from build123d import *

# Parameters (mm, degrees)
SKETCH_1_R               = 8.5
EXTRUDE_1_DEPTH          = 1.2
SKETCH_2_R               = 8.5
SKETCH_2_R_2             = 7
EXTRUDE_2_DEPTH          = 5.5
SKETCH_3_R               = 7
SKETCH_3_R_2             = 6.5
EXTRUDE_3_DEPTH          = 0.3
SKETCH_4_W               = 1
SKETCH_4_H               = 4.082242853
CUT_EXTRUDE_1_DEPTH      = 5
PATTERN_CIRCULAR_1_COUNT = 8
SKETCH_5_W               = 1.4
SKETCH_5_H               = 2.4
EXTRUDE_4_DEPTH          = 1.7


with BuildPart() as part:
    # Эскиз1 → Бобышка-Вытянуть1 (new body)
    with BuildSketch(Plane(origin=(0, 0, 0), x_dir=(1, 0, 0), z_dir=(0, 1, 0))):
        with Locations(Location((0, 0, 0), (0, 0, 270))):
            Circle(SKETCH_1_R)
    extrude(amount=EXTRUDE_1_DEPTH)

    # Эскиз2 → Бобышка-Вытянуть2 (add)
    with BuildSketch(Plane(origin=(0, 1.2, 0), x_dir=(1, 0, 0), z_dir=(0, 1, 0))):
        with Locations(Location((0, 0, 0), (0, 0, 270))):
            Circle(SKETCH_2_R)
        with Locations(Location((0, 0, 0), (0, 0, 270))):
            Circle(SKETCH_2_R_2, mode=Mode.SUBTRACT)
    extrude(amount=EXTRUDE_2_DEPTH)

    # Эскиз3 → Бобышка-Вытянуть3 (add)
    with BuildSketch(Plane(origin=(0, 1.2, 0), x_dir=(1, 0, 0), z_dir=(0, 1, 0))):
        with Locations(Location((0, 0, 0), (0, 0, 270))):
            Circle(SKETCH_3_R)
        with Locations(Location((0, 0, 0), (0, 0, 270))):
            Circle(SKETCH_3_R_2, mode=Mode.SUBTRACT)
    extrude(amount=EXTRUDE_3_DEPTH)

    # Эскиз4 → Вырез-Вытянуть1 (cut)
    with BuildSketch(Plane(origin=(0, 6.7, 0), x_dir=(1, 0, 0), z_dir=(0, 1, 0))):
        with Locations((0, 7.692447021)):
            Rectangle(SKETCH_4_W, SKETCH_4_H)
    cut_extrude_1 = extrude(amount=-CUT_EXTRUDE_1_DEPTH, mode=Mode.SUBTRACT)

    # Круговой массив1: Вырез-Вытянуть1 ×8 about axis
    pattern_circular_1_axis = Axis((0, 0, 0), (0, 1, 0))
    for i in range(1, PATTERN_CIRCULAR_1_COUNT):
        add(cut_extrude_1.rotate(pattern_circular_1_axis, i * 360 / PATTERN_CIRCULAR_1_COUNT), mode=Mode.SUBTRACT)

    # Эскиз5 → Бобышка-Вытянуть4 (add)
    with BuildSketch(Plane.XZ):
        with BuildLine():
            Line((-11.124038405, -2.5), (-8.124038405, -2.5))
            ThreePointArc((-8.124038405, -2.5), (-8.5, 0), (-8.124038405, 2.5))
            Line((-8.124038405, 2.5), (-11.124038405, 2.5))
            ThreePointArc((-11.124038405, 2.5), (-11.831145186, 2.207106781), (-12.124038405, 1.5))
            Line((-12.124038405, 1.5), (-12.124038405, -1.5))
            ThreePointArc((-12.124038405, -1.5), (-11.831145186, -2.207106781), (-11.124038405, -2.5))
        make_face()
        with Locations((-10.124038405, 0)):
            Rectangle(SKETCH_5_W, SKETCH_5_H, mode=Mode.SUBTRACT)
    extrude(amount=-EXTRUDE_4_DEPTH)


solid = part.part
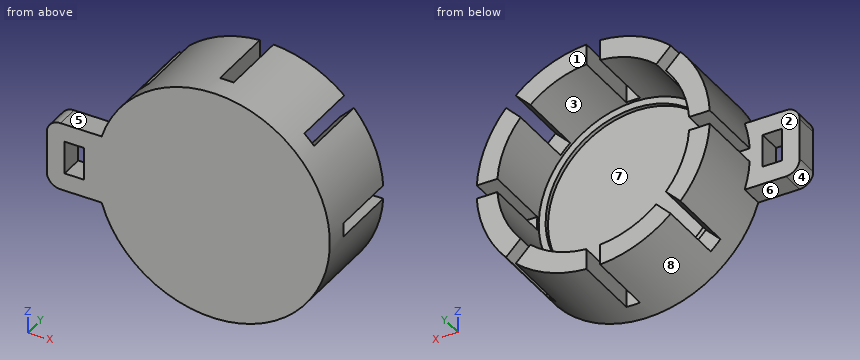
Read the model definition and answer for the solid it produces. Units are mm, in the model's axes. Face numbers are marked on the shaded views. A direction names the side the tool comes from. Give positions to 0.01 mm unless a question says otherwise; leave off trailing zeros. Write each loop counter-clockwise with the first axis right and the second up, starting at its lowest first coordinate (ties: lowest second). Pieces come first, ordered by that corner, then holes. Notation, with made-up numbers: (-34, -16.5) -> (-10, -16.5) arc R25 ccw to (-10, 3.5) -> close; hole circle Ø5 at (86.5, 8.5). An arc over 180 degrees is marked (long way). Answer as a JSON object with one key per item and string values. Group by question number.
1) The mould has two halves that part along X. Classify the marked faces 6, 7 and 8: +X half, -X half, draft (parallel to the pull), parting line (faces both ways), or undercut.
2) Consider L1, parallel to X at y = 1.4, z = 0; L2, parallel to Y at x = 2.25, z = -1.75; L3, parallel to X at y = 5, z = 5. Determine where each line is inside the solid, lowest interval first. Write a range as from..to.
3) Each of these flat-tipped pins is pushed along its axis until it touches: P1, Ø2, axis at x = -5.5, y = 0.5, coming from the +Z side; P2, Ø2, axis at x = -10, y = 2.5, coming from the +Z side; P3, Ø1.5, axis at x = -8, y = 3, coming from the +Z side; P4, Ø0.5, axis at x = 6, z = -5.5, coming from the +Y side. Where does it stop, or does it pass through?
4) Find section D-D (x = 0). Write down the section's boundary in (y, z), and give its area (3 significant figures).
5) Find section C-C (z = 0). Write down the section's boundary in (x, y).
6) A tool of negligible diameter and unlimited length cuts with its end or side. For the marked faces 1, 2, 3, 4 and 5, from which of +Z, -Z, +X, -X, +Y, -Y can it reach the whole face along a straight path? Write none if from no direction.
7) Find section B-B (x = -10.5). Write down the section's boundary in (y, z).
8) Find section A-A (y = 3.5). Count the separate pieces of the cut face and the enclosed holes in it, and give its area (3 significant figures).
Values follow:
{
 "1": {"face 6": "draft", "face 7": "undercut", "face 8": "parting line"},
 "2": {"L1": "x = -12.12..-10.82, -9.42..-6.5, 6.5..8.5", "L2": "y = 0..1.2", "L3": "x = -6.87..-5.71, 5.71..6.87"},
 "3": {"P1": "stops at z = 7.21", "P2": "stops at z = 2.5", "P3": "stops at z = 4.44", "P4": "stops at y = 6.7"},
 "4": {"outline": "(0, -8.5) -> (1.7, -8.5) -> (1.7, -7) -> (1.5, -7) -> (1.5, -6.5) -> (1.2, -6.5) -> (1.2, 6.5) -> (1.5, 6.5) -> (1.5, 7) -> (1.7, 7) -> (1.7, 8.5) -> (0, 8.5) -> close", "area": "22.2 mm2"},
 "5": {"outline": "(-12.12, 0) -> (-10.82, 0) -> (-10.82, 1.7) -> (-12.12, 1.7) -> close; (-9.42, 0) -> (8.5, 0) -> (8.5, 1.7) -> (7, 1.7) -> (7, 1.5) -> (6.5, 1.5) -> (6.5, 1.2) -> (-6.5, 1.2) -> (-6.5, 1.5) -> (-7, 1.5) -> (-7, 1.7) -> (-9.42, 1.7) -> close"},
 "6": {"face 1": "+Z, -Z, +X, -X, +Y", "face 2": "-X, +Y", "face 3": "+Y", "face 4": "-Z, -X, +Y, -Y", "face 5": "+Z, -X, +Y, -Y"},
 "7": {"outline": "(0, -2.5) -> (1.7, -2.5) -> (1.7, -1.2) -> (0, -1.2) -> close; (0, 1.2) -> (1.7, 1.2) -> (1.7, 2.5) -> (0, 2.5) -> close"},
 "8": {"separate pieces": "8", "enclosed holes": "0", "area": "61.0 mm2"}
}
